Read the model definition and answer for the solid it produces. Units are mm, in the model's axes. Face numbers are marked on the shaded views. A direction names the side the tool comes from. Give positions to 0.01 mm unless a question says otherwise; leave off trailing zeros. Order: outer loops, then holes, each group sorted by start corner. A loop starts at its lowest first (then second) coordinate and runs counter-clockwise, first axis right, second up. Notation, with made-up numbers: (12.5, 35) -> (48.5, 35) arc R16 ccw to (48.5, 62) -> close; hole circle Ø11 at (-30.5, -2.75). An arc over 180 degrees is marked (long way). Answer as CSV lines item,"result". Start each with the question number.
1) Straight lines are drawn through the part: L1, parallel to Z at x = 0, y = -1.5; L2, parallel to Z at x = 2, y = 0.25 (3 decimals); L3, parallel to Y at x = 0, z = 23.75. For each, find the intervals that lie inside material, in ascending order. Write a range as from..to.
2) Find section A-A (x = 0). Determine the outline of the cut face in (y, z) (1 decimal), and give its area (3 significant figures).
3) Flat-ended cylindrical pins translate along their axes: pin 1 Ø1.3 at (y, z) = (1, 27.5) entering from -X; pin 2 Ø0.9 at (x, z) = (1, 27.5) entering from +Y; pin 3 Ø1.3 at (x, y) = (-3, -1.5) entering from -Z (3 decimals). Find the tip coordinate at first contact, or state that the pin passes through.
4) Find section B-B (z = 14). Determine the outline of the cut face in (x, y), and give its area (3 significant figures).
5) For the marked faces 1, 2 and 3, determine the directions among +Z, -Z, +X, -X, +Y, -Y from which every point of the face is accessible in a straight line to the end or side of a thin tool.
Autodesk Inventor part; units mm, degrees
ref_plane "Work Plane1" through (0, 0, 28.067) normal (0, 0, 1) x (1, 0, 0)
ref_plane "YZ Plane" through (0, 0, 0) normal (1, 0, 0) x (0, 1, 0)
ref_plane "XZ Plane" through (0, 0, 0) normal (0, 1, 0) x (-1, 0, 0)
sketch "Sketch1" plane through (0, 0, 0) normal (0, 0, 1) x (1, 0, 0)
  circle A0 centre (0, 0) radius 1.9685
  dimension "d0" = 3.937
sketch "Sketch1 outline for Extrusion1" plane through (0, 0, 0) normal (0, 0, 1) x (1, 0, 0)
  circle A0 centre (0, 0) radius 1.9685
extrude "Extrusion1" add sketch "Sketch1 outline for Extrusion1" along normal blind 24.765
sketch "Sketch2" plane through (0, 0, 24.765) normal (0, 0, 1) x (1, 0, 0)
  circle A0 centre (0, 0) radius 1.9685
  line L0 (-1.397, 3.68081) -> (-1.397, 1.386861)
  line L1 (1.397, 3.68081) -> (1.397, 1.386861)
  line L2 (1.397, -3.68081) -> (1.397, -1.386861)
  line L3 (-1.397, -3.68081) -> (-1.397, -1.386861)
  arc A1 (1.397, 3.68081) -> (-1.397, 3.68081) centre (0, 0) ccw
  arc A2 (-1.397, -3.68081) -> (1.397, -3.68081) centre (0, 0) ccw
  arc A3 (-1.397, 1.386861) -> (-1.397, -1.386861) centre (0, 0) ccw
  arc A4 (1.397, -1.386861) -> (1.397, 1.386861) centre (0, 0) ccw
  point P0 (0, 1.9685)
  point P1 (0, -1.9685)
  point P2 (1.397, 1.9685)
  point P3 (-1.397, 1.9685)
  point P4 (1.397, -1.9685)
  point P5 (-1.397, -1.9685)
  dimension "d6" = 1.397
  dimension "d7" = 1.397
  dimension "d8" = 1.397
  dimension "d9" = 1.397
sketch "Sketch2 outline for Extrusion2" plane through (0, 0, 24.765) normal (0, 0, 1) x (1, 0, 0)
  arc A0 (1.397, 3.68081) -> (-1.397, 3.68081) centre (0, 0) ccw
  line L0 (-1.397, 3.68081) -> (-1.397, 1.386861)
  arc A1 (-1.397, 1.386861) -> (-1.397, -1.386861) centre (0, 0) ccw
  line L1 (-1.397, -1.386861) -> (-1.397, -3.68081)
  arc A2 (-1.397, -3.68081) -> (1.397, -3.68081) centre (0, 0) ccw
  line L2 (1.397, -3.68081) -> (1.397, -1.386861)
  arc A3 (1.397, -1.386861) -> (1.397, 1.386861) centre (0, 0) ccw
  line L3 (1.397, 1.386861) -> (1.397, 3.68081)
extrude "Extrusion2" add sketch "Sketch2 outline for Extrusion2" along normal blind 1.27
sketch "Sketch3" plane through (0, 0, 26.035) normal (0, 0, 1) x (1, 0, 0)
  arc A0 (1.397, 3.68081) -> (-1.397, 3.68081) centre (0, 0) ccw
  circle A1 centre (0, 0) radius 3.937
sketch "Sketch3 outline for Extrusion3" plane through (0, 0, 26.035) normal (0, 0, 1) x (1, 0, 0)
  circle A0 centre (0, 0) radius 3.937
extrude "Extrusion3" add sketch "Sketch3 outline for Extrusion3" along normal blind 1.27
ref_plane "Work Plane1" through (0, 0, 28.067) normal (0, 0, 1) x (1, 0, 0)
sketch "Sketch4" plane through (0, 0, 28.067) normal (0, 0, 1) x (1, 0, 0)
  circle A0 centre (0, 0) radius 0.127
  dimension "d15" = 0.254
sketch "Sketch4 outline for Loft1" plane through (0, 0, 28.067) normal (0, 0, 1) x (1, 0, 0)
  circle A0 centre (0, 0) radius 0.127
loft "Loft1" add profiles "Sketch4 outline for Loft1" section 2 edges at (-3.937, 0, 27.305)
sketch "Sketch5" plane through (0, 0, 28.067) normal (0, 0, 1) x (1, 0, 0)
  circle A0 centre (0, 0) radius 0.127
  line L0 (-0.508, 2.032) -> (0.508, 2.032)
  line L1 (0.508, 2.032) -> (0.508, 0.508)
  line L2 (0.508, 0.508) -> (2.032, 0.508)
  line L3 (2.032, 0.508) -> (2.032, -0.508)
  line L4 (2.032, -0.508) -> (0.508, -0.508)
  line L5 (0.508, -0.508) -> (0.508, -2.032)
  line L6 (0.508, -2.032) -> (-0.508, -2.032)
  line L7 (-0.508, -2.032) -> (-0.508, -0.508)
  line L8 (-0.508, -0.508) -> (-2.032, -0.508)
  line L9 (-2.032, -0.508) -> (-2.032, 0.508)
  line L10 (-2.032, 0.508) -> (-0.508, 0.508)
  line L11 (-0.508, 0.508) -> (-0.508, 2.032)
  dimension "d22" = 0.508
  dimension "d23" = 0.508
  dimension "d24" = 0.508
  dimension "d25" = 0.508
  dimension "d26" = 2.032
  dimension "d27" = 2.032
  dimension "d28" = 2.032
  dimension "d29" = 2.032
  dimension "d30" = 2.032
  dimension "d31" = 2.032
  dimension "d32" = 2.032
  dimension "d33" = 2.032
sketch "Sketch5 outline for Extrusion4" plane through (0, 0, 28.067) normal (0, 0, 1) x (1, 0, 0)
  line L0 (2.032, 0.508) -> (0.508, 0.508)
  line L1 (2.032, -0.508) -> (2.032, 0.508)
  line L2 (0.508, -0.508) -> (2.032, -0.508)
  line L3 (0.508, -2.032) -> (0.508, -0.508)
  line L4 (-0.508, -2.032) -> (0.508, -2.032)
  line L5 (-0.508, -0.508) -> (-0.508, -2.032)
  line L6 (-2.032, -0.508) -> (-0.508, -0.508)
  line L7 (-2.032, 0.508) -> (-2.032, -0.508)
  line L8 (-0.508, 0.508) -> (-2.032, 0.508)
  line L9 (-0.508, 2.032) -> (-0.508, 0.508)
  line L10 (0.508, 2.032) -> (-0.508, 2.032)
  line L11 (0.508, 0.508) -> (0.508, 2.032)
extrude "Extrusion4" cut sketch "Sketch5 outline for Extrusion4" against normal blind 1.27
thread "Thread1"
properties part number "Prop Screw" material "Stainless Steel"
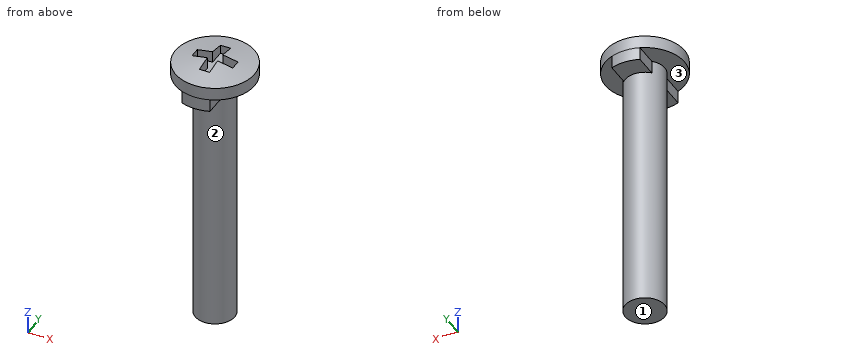
Findings below:
1,L1,"0..26.8"
1,L2,"26.035..26.797"
1,L3,"-1.97..1.97"
2,outline,"(-3.9, 24.8) -> (-2, 24.8) -> (-2, 0) -> (2, 0) -> (2, 24.8) -> (3.9, 24.8) -> (3.9, 27.3) -> (2, 27.7) -> (2, 26.8) -> (-2, 26.8) -> (-2, 27.7) -> (-3.9, 27.3) -> close"
2,area,"116 mm²"
3,pin 1,"x = -3.92"
3,pin 2,"y = 3.89"
3,pin 3,"z = 26.035"
4,outline,"circle Ø3.94 at (0, 0)"
4,area,"12.2 mm²"
5,face 1,"-Z, +X, -X, +Y, -Y"
5,face 2,"-Z"
5,face 3,"-Z, -X"
